Can you work these out from the model? Positions are in its coordinate system, mm. A direction names the side the tool comes from. Round coordinates to 2 decimals unless told otherwise and drop trailing zeros. Write each loop counter-clockwise with the first axis right and the second up, starting at its lowest first coordinate (ties: lowest second). Pieces come first, ordered by that corner, then holes. Notation, with made-up numbers: M 78,81 L 95,81 A28 cw 95,100 Z; hole C 3.5,-21.75 d7. An arc over 180 degrees is marked long. Answer in a Markdown table with one row per item. Add a question column.
(1) If I drill on probe 1 along X at (y, z) = (1.25, 1.1); probe 2 along X at (y, z) = (0.75, -0.35); probe 3 along Z at (x, y) = (0.3, -3), over which ranges is the centre line in solid material (lowest first)?
(2) For faces 1 (the face through (-1.683, 0.266, 1.291)), 2 (the face through (-0.917, 0.934, 0.006)), which set-ups out of +Z, -Z, +X, -X, +Y, -Y let a thin tool reach every point of the face, with its end or its side?
(3) Suppose I cut it at A-A, the plane y = -2.5. Write out the boundary of the cut face in (x, z), then the cut area to 3 significant figures.
(4) I'm going to push flat-ended pins straight in: pin 1 (0.8 mm diameter, centred on x = -1, y = 1, fed in from -Z); pin 2 (1.1 mm diameter, centred on y = 1, z = -1, fed in from -X); pin 3 (1 mm diameter, centred on x = -0.5, z = 1.5, fed in from +Y); pin 4 (1.5 mm diameter, centred on y = 1, z = -0.5, fed in from +X). Where does each tip first touch, or does it pass through?
(5) If we mould it in two halves opening along X, with no side actions, what happens to faces 3 (the face through (0.931, 0.947, 0.006)), 4 (the face through (-1, 0, -1)), 5 (the face through (-0.8, 1.1, 0.394)), 6 (the face through (1.04, -2.28, 0.33))? For each: released by +X, released by -X, zero draft, split by the parting line, or undercut.
Autodesk Inventor part; units mm, degrees
ref_plane "YZ Plane" through (0, 0, 0) normal (1, 0, 0) x (0, 1, 0)
ref_plane "XZ Plane" through (0, 0, 0) normal (0, 1, 0) x (-1, 0, 0)
ref_plane "XY Plane" through (0, 0, 0) normal (0, 0, 1) x (1, 0, 0)
sketch "Sketch1" plane through (0, 0, 0) normal (0, 0, 1) x (1, 0, 0)
  line L0 (0, -5.4574) -> (0, 4.0933)
  line L1 (2.1209, 0) -> (2.1209, 0.5237)
  arc A0 (2.1209, 0.5237) -> (1.5692, 1.3462) centre (1.2319, 0.5237) ccw
  arc A1 (1.5692, 1.3462) -> (0.7645, 1.5048) centre (0.7645, -0.6161) ccw
  line L2 (0.7645, 1.5048) -> (0, 1.5048)
  line L3 (2.1209, 0) -> (1.0922, 0)
  line L4 (1.0922, 0) -> (1.0922, -4.7752)
  line L5 (1.0922, -4.7752) -> (0, -4.7752)
  point P0 (0, 0)
  dimension "d0" = 2.1844
  dimension "d1" = 4.2418
  dimension "d2" = 0.889
  dimension "d3" = 2.1209
  dimension "d4" = 4.7752
  dimension "d6" = 1.5291
  dimension "d8" = 1.3462
revolve "Revolution1" add sketch "Sketch1" angle 360 about axis through (0, -10, 0) along (0, 1, 0)
sketch "Sketch2" plane through (0, 0, 0) normal (0, 0, 1) x (1, 0, 0)
  line L0 (0, 0.1586) -> (-1.5907, 1.5048)
  line L1 (-1.5907, 1.5048) -> (1.5907, 1.5048)
  line L2 (1.5907, 1.5048) -> (0, 0.1586)
  line L3 (0, 0.0835) -> (0, 2.5016)
  line L4 (-0.7645, 1.5048) -> (0.7645, 1.5048)
  dimension "d9" = 3.1814
  dimension "d22" = 1.3462
extrude "Extrusion1" cut sketch "Sketch2" against normal mid plane 0.7874
sketch "Sketch3" plane through (0, 0, 0) normal (1, 0, 0) x (0, 1, 0)
  line L0 (1.5048, 1.5907) -> (1.5048, -1.5907)
  line L1 (1.5048, -1.5907) -> (0.1586, 0)
  line L2 (0.1586, 0) -> (1.5048, 1.5907)
  point P0 (1.5048, 0)
  point P1 (1.5048, 0)
  point P2 (1.5048, 0)
  dimension "d12" = 3.1814
extrude "Extrusion2" cut sketch "Sketch3" against normal mid plane 0.7874
sketch "Sketch4" plane through (-0.6554, 1.5048, 0.3937) normal (0, 1, 0) x (1, 0, 0)
  arc A0 (0, 0) -> (0.2617, -0.2617) centre (0.6554, 0.3937) ccw
  circle A1 centre (0.6554, 0.3937) radius 0.7645
  dimension "d17" = 1.5291
extrude "Extrusion3" cut sketch "Sketch4" against normal blind 0.7645 draft -30
thread "Thread1"
chamfer "Chamfer1" distance 0.2731 angle 45 1 edges at (-1.0922, -4.7752, 0)
equation "\"d0\" = Dia"
equation "\"d1\" = HeadDia"
equation "\"d2\" = HeadRad"
equation "\"d3\" = 0.5 * d1"
equation "\"d4\" = ShankLength"
equation "\"d6\" = 0.7 * d0"
equation "\"d8\" = HeadHeight"
equation "\"d9\" = 0.75 * d1"
equation "\"d22\" = HeadHeight"
equation "\"d10\" = SlotW"
equation "\"d12\" = d9"
equation "\"d13\" = SlotW"
equation "\"d17\" = d6"
equation "\"d15\" = 0.5 * d6"
equation "\"d18\" = ThreadLength"
equation "\"d20\" = 0.125 * Dia"
equation "\"d21\" = 0.125 * Dia"
equation "\"Dia\" = 2.1844"
equation "\"ShankLength\" = 4.7752"
equation "\"HeadDia\" = 4.2418"
equation "\"HeadRad\" = 0.889"
equation "\"SlotW\" = 0.7874"
equation "\"SlotD\" = 0.7874"
equation "\"HeadHeight\" = 1.3462"
equation "\"ThreadLength\" = 4.5466"
properties part number "Phillips Pan Head Machine Screw Inch" material "Steel, High Strength Low Alloy"
Calculated:
| question | item | result |
|---|---|---|
| 1 | probe 1 | -1.35 to -0.39, 0.39 to 1.35 |
| 1 | probe 2 | -2.06 to -0.7, 0.7 to 2.06 |
| 1 | probe 3 | -1.05 to 1.05 |
| 2 | face 1 | +Y, -Y |
| 2 | face 2 | +Y |
| 3 | outline | C 0,0 d2.18 |
| 3 | area | 3.75 mm² |
| 4 | pin 1 | z = -1.98 |
| 4 | pin 2 | x = -2.03 |
| 4 | pin 3 | y = 1.48 |
| 4 | pin 4 | x = 2.12 |
| 5 | face 3 | undercut |
| 5 | face 4 | zero draft |
| 5 | face 5 | undercut |
| 5 | face 6 | split by the parting line |
